```python
from build123d import *

# Parameters (mm, degrees)
SKETCH1_R           = 102.5
SKETCH1_R_2         = 60
BOSS_EXTRUDE1_DEPTH = 6
SKETCH2_R           = 4
CUT_EXTRUDE1_DEPTH  = 146.081011852
CIRPATTERN1_COUNT   = 20
SKETCH4_OUTSIDE_W   = 264.996
SKETCH4_OUTSIDE_H   = 264.996
SKETCH4_OUTSIDE_R   = 86
CUT_EXTRUDE3_DEPTH  = 146.081011852
CUT_EXTRUDE4_DEPTH  = 10
BOSS_EXTRUDE2_DEPTH = 6
FILLET1_R           = 6


with BuildPart() as part:
    # Sketch1 → Boss-Extrude1 (new body)
    with BuildSketch(Plane(origin=(0, 0, 0), x_dir=(1, 0, 0), z_dir=(0, 1, 0))):
        with Locations(Location((0, 0, 0), (0, 0, 270))):
            Circle(SKETCH1_R)
        with Locations(Location((0, 0, 0), (0, 0, 270))):
            Circle(SKETCH1_R_2, mode=Mode.SUBTRACT)
    extrude(amount=BOSS_EXTRUDE1_DEPTH)

    # Sketch2 → Cut-Extrude1 (cut, through all)
    with BuildSketch(Plane(origin=(0, 6, 0), x_dir=(1, 0, 0), z_dir=(0, 1, 0))):
        with Locations(Location((0, 70, 0), (0, 0, 270))):
            Circle(SKETCH2_R)
    cut_extrude1 = extrude(amount=-CUT_EXTRUDE1_DEPTH, mode=Mode.SUBTRACT)

    # CirPattern1: Cut-Extrude1 ×20 about axis
    cirpattern1_axis = Axis((0, 0, 0), (0, 1, 0))
    for i in range(1, CIRPATTERN1_COUNT):
        add(cut_extrude1.rotate(cirpattern1_axis, i * 360 / CIRPATTERN1_COUNT), mode=Mode.SUBTRACT)

    # Sketch4 outside → Cut-Extrude3 (cut, through all)
    with BuildSketch(Plane(origin=(0, 6, 0), x_dir=(1, 0, 0), z_dir=(0, 1, 0))):
        Rectangle(SKETCH4_OUTSIDE_W, SKETCH4_OUTSIDE_H)
        with Locations(Location((0, 0, 0), (0, 0, 270))):
            Circle(SKETCH4_OUTSIDE_R, mode=Mode.SUBTRACT)
    extrude(amount=-CUT_EXTRUDE3_DEPTH, mode=Mode.SUBTRACT)

    # Sketch5 → Cut-Extrude4 (cut)
    with BuildSketch(Plane(origin=(0, 6, 0), x_dir=(1, 0, 0), z_dir=(0, 1, 0))):
        with BuildLine():
            ThreePointArc((46.694681279, 42.270046437), (48.541019662, 35.267115138), (54.63065317, 31.347118204))
            ThreePointArc((54.63065317, 31.347118204), (57.394464692, 29.243940421), (57.471443608, 25.771753046))
            ThreePointArc((57.471443608, 25.771753046), (57.063390978, 18.541019662), (61.643630936, 12.931080792))
            ThreePointArc((61.643630936, 12.931080792), (63.622254217, 10.076775126), (62.622500611, 6.750740904))
            ThreePointArc((62.622500611, 6.750740904), (60, 0), (62.622500611, -6.750740904))
            ThreePointArc((62.622500611, -6.750740904), (63.622254217, -10.076775126), (61.643630936, -12.931080792))
            ThreePointArc((61.643630936, -12.931080792), (57.063390978, -18.541019662), (57.471443608, -25.771753046))
            ThreePointArc((57.471443608, -25.771753046), (57.394464692, -29.243940421), (54.63065317, -31.347118204))
            ThreePointArc((54.63065317, -31.347118204), (48.541019662, -35.267115138), (46.694681279, -42.270046437))
            ThreePointArc((46.694681279, -42.270046437), (45.548505072, -45.548505072), (42.270046437, -46.694681279))
            ThreePointArc((42.270046437, -46.694681279), (35.267115138, -48.541019662), (31.347118204, -54.63065317))
            ThreePointArc((31.347118204, -54.63065317), (29.243940421, -57.394464692), (25.771753046, -57.471443608))
            ThreePointArc((25.771753046, -57.471443608), (18.541019662, -57.063390978), (12.931080792, -61.643630936))
            ThreePointArc((12.931080792, -61.643630936), (10.076775126, -63.622254217), (6.750740904, -62.622500611))
            ThreePointArc((6.750740904, -62.622500611), (0, -60), (-6.750740904, -62.622500611))
            ThreePointArc((-6.750740904, -62.622500611), (-10.076775126, -63.622254217), (-12.931080792, -61.643630936))
            ThreePointArc((-12.931080792, -61.643630936), (-18.541019662, -57.063390978), (-25.771753046, -57.471443608))
            ThreePointArc((-25.771753046, -57.471443608), (-29.243940421, -57.394464692), (-31.347118204, -54.63065317))
            ThreePointArc((-31.347118204, -54.63065317), (-35.267115138, -48.541019662), (-42.270046437, -46.694681279))
            ThreePointArc((-42.270046437, -46.694681279), (-45.548505072, -45.548505072), (-46.694681279, -42.270046437))
            ThreePointArc((-46.694681279, -42.270046437), (-48.541019662, -35.267115138), (-54.63065317, -31.347118204))
            ThreePointArc((-54.63065317, -31.347118204), (-57.394464692, -29.243940421), (-57.471443608, -25.771753046))
            ThreePointArc((-57.471443608, -25.771753046), (-57.063390978, -18.541019662), (-61.643630936, -12.931080792))
            ThreePointArc((-61.643630936, -12.931080792), (-63.622254217, -10.076775126), (-62.622500611, -6.750740904))
            ThreePointArc((-62.622500611, -6.750740904), (-60, 0), (-62.622500611, 6.750740904))
            ThreePointArc((-62.622500611, 6.750740904), (-63.622254217, 10.076775126), (-61.643630936, 12.931080792))
            ThreePointArc((-61.643630936, 12.931080792), (-57.063390978, 18.541019662), (-57.471443608, 25.771753046))
            ThreePointArc((-57.471443608, 25.771753046), (-57.394464692, 29.243940421), (-54.63065317, 31.347118204))
            ThreePointArc((-54.63065317, 31.347118204), (-48.541019662, 35.267115138), (-46.694681279, 42.270046437))
            ThreePointArc((-46.694681279, 42.270046437), (-45.548505072, 45.548505072), (-42.270046437, 46.694681279))
            ThreePointArc((-42.270046437, 46.694681279), (-35.267115138, 48.541019662), (-31.347118204, 54.63065317))
            ThreePointArc((-31.347118204, 54.63065317), (-29.243940421, 57.394464692), (-25.771753046, 57.471443608))
            ThreePointArc((-25.771753046, 57.471443608), (-18.541019662, 57.063390978), (-12.931080792, 61.643630936))
            ThreePointArc((-12.931080792, 61.643630936), (-10.076775126, 63.622254217), (-6.750740904, 62.622500611))
            ThreePointArc((-6.750740904, 62.622500611), (0, 60), (6.750740904, 62.622500611))
            ThreePointArc((6.750740904, 62.622500611), (10.076775126, 63.622254217), (12.931080792, 61.643630936))
            ThreePointArc((12.931080792, 61.643630936), (18.541019662, 57.063390978), (25.771753046, 57.471443608))
            ThreePointArc((25.771753046, 57.471443608), (29.243940421, 57.394464692), (31.347118204, 54.63065317))
            ThreePointArc((31.347118204, 54.63065317), (35.267115138, 48.541019662), (42.270046437, 46.694681279))
            ThreePointArc((42.270046437, 46.694681279), (45.548505072, 45.548505072), (46.694681279, 42.270046437))
        make_face()
    extrude(amount=-CUT_EXTRUDE4_DEPTH, mode=Mode.SUBTRACT)

    # Sketch6 → Boss-Extrude2 (add)
    with BuildSketch(Plane(origin=(0, 6, 0), x_dir=(1, 0, 0), z_dir=(0, 1, 0))):
        with BuildLine():
            Line((-17.398199941, -88.302336542), (8.989447841, -85.528883002))
            ThreePointArc((8.989447841, -85.528883002), (-74.100107798, 43.648299215), (79.163417397, 33.60287705))
            Line((79.163417397, 33.60287705), (82.845436811, 35.165801564))
            ThreePointArc((82.845436811, 35.165801564), (-69.870812829, 56.728031119), (-17.398199941, -88.302336542))
        make_face()
    extrude(amount=-BOSS_EXTRUDE2_DEPTH)

    # Fillet1
    # the kernel refuses this fillet: 6 mm, written as the material it adds along each edge
    with BuildSketch(Plane(origin=(79.163417397, 6, -33.60287705), x_dir=(0.36192981714556505, 0, 0.9322053461877259), z_dir=(0, -1, 0))) as fillet1_piece_1:
        with BuildLine():
            CenterArc((5.532861862, -5.997100749), FILLET1_R, 91.781239909, 68.757327573)
            Line((-0.124333974, -3.998067166), (-0.237477891, -3.958086494))
            ThreePointArc((-0.237477891, -3.958086494), (-0.182109002, -1.995303564), (-0.119942015, 0.003730019))
            Line((-0.119942015, 0.003730019), (0.003730019, 0.119942015))
            ThreePointArc((0.003730019, 0.119942015), (2.67318045, 0.078444066), (5.342630881, 0.119942015))
            Line((5.342630881, 0.119942015), (5.346360901, 0))
        make_face()
    extrude(amount=6)


solid = part.part
```
Could you check a few things on this model? Use its own coordinates, in mm. Coordinates: 2 decimals unless noted, no trailing zeros. Write each loop counter-clockwise with the first axis right and the second up, starting at its lowest first coordinate (ties: lowest second). Pieces come first, ordered by that corner, then holes. Notation, with made-up numbers: (19.25, -1) -> (28.25, -1) arc R20 cw to (28.25, 34) -> close; hole circle Ø5 at (29, 12). An arc over 180 degrees is marked (long way). Return JSON: item names as keys, results as strings.
(1) I'm going to push flat-ended pins straight in: pin 1 (9 mm diameter, centred on x = -41.14, z = -56.63, fed in from -Y); pin 2 (1.5 mm diameter, centred on x = 6, y = 3, fed in from -Z); pin 3 (3 mm diameter, centred on y = 5.5, z = -6.5, fed in from +X). Where does each tip first touch, or does it pass through?
Numbers:
{"pin 1": "stops at y = 0", "pin 2": "stops at z = -89.85", "pin 3": "stops at x = 85.85"}
(2) Imagine slicing it at A-A, the plane z = 0. Please give me the cut outline in (x, y).
Numbers:
{"outline": "(-90, 0) -> (-74, 0) -> (-74, 6) -> (-90, 6) -> close; (-66, 0) -> (-60, 0) -> (-60, 6) -> (-66, 6) -> close; (60, 0) -> (66, 0) -> (66, 6) -> (60, 6) -> close; (74, 0) -> (86, 0) -> (86, 6) -> (74, 6) -> close"}
(3) Imagine slicing it at B-B, the plane x = 0. Please give me the cut outline in (y, z), then the cut area to 3 significant figures.
Numbers:
{"outline": "(0, -90) -> (6, -90) -> (6, -74) -> (0, -74) -> close; (0, -66) -> (6, -66) -> (6, -60) -> (0, -60) -> close; (0, 60) -> (6, 60) -> (6, 66) -> (0, 66) -> close; (0, 74) -> (6, 74) -> (6, 86.47) -> (0, 86.47) -> close", "area": "243 mm2"}
(4) Imagine slicing it at D-D, the plane y = 2.85. Count the separate pieces of the cut face and the enclosed holes in it, then the cut area to 3 significant figures.
Numbers:
{"separate pieces": "1", "enclosed holes": "21", "area": "11,700 mm2"}
(5) I need wall thicknesses on L1, parallel to X at y = 5.2, z = -65; L2, parallel to Z at x = -63, y = 5.6; L3, parallel to X at y = 4.7, z = 69. Which ranges of each line are inside material? Lowest first, please.
Numbers:
{"L1": "x = -62.25 to -25.31, -17.95 to 17.95, 25.31 to 62.25", "L2": "z = -64.27 to -23.43, -19.83 to -11.67, -7.23 to 7.23, 11.67 to 19.83, 23.43 to 64.27", "L3": "x = -57.78 to -24.81, -18.45 to -3.87, 3.87 to 18.45, 24.81 to 51.33"}
(6) Imagine slicing it at C-C, the plane z = 35. Please give me the cut outline in (x, y), then the cut area to 3 significant figures.
Numbers:
{"outline": "(-82.92, 0) -> (-48.74, 0) -> (-48.74, 6) -> (-82.92, 6) -> close; (48.74, 0) -> (78.56, 0) -> (78.56, 6) -> (48.74, 6) -> close", "area": "384 mm2"}
(7) We'd pull the mould along Z, two halves only. Please class faces 1 (the cylindrical face through (-57.096, 3.042, -18.443)), 2 (the flat face through (-57, 0, 21)): +Z half, -Z half, draft (parallel to the pull), parting line (faces both ways), or undercut.
Numbers:
{"face 1": "undercut", "face 2": "draft"}
